Geometry: final body of the model. Coordinates: model frame, mm. A direction names the side the tool comes from. Coordinates: 2 decimals unless noted, no trailing zeros. Write each loop counter-clockwise with the first axis right and the second up, starting at its lowest first coordinate (ties: lowest second). Pieces come first, ordered by that corner, then holes. Notation, with made-up numbers: M 15,86 L 33,86 A26 ccw 33,124 Z; hole C 53,13 d8. An arc over 180 degrees is marked long. Write item = value, one per line. Start each with the question number.
Item 1: Reachability of faces 1 (the flat face through (0, 0, -9)), 2 (the cylindrical face through (-1.22, -15.16, -4.09)), 3 (the cylindrical face through (-4.09, -15.05, -1.23)), 4 (the cylindrical face through (2.26, 1.29, -1.18)), 5 (the flat face through (0, 2, -9)) from +Z, -Z, +X, -X, +Y, -Y: full face, straight path, thin tool, end or side. Return the list, or none.
Item 2: Section B-B on z = 0. Give the number of separate pieces and of enclosed holes in the cut face, plus the area to 3 significant figures.
Item 3: Ray query, L1, parallel to Y at x = -5, z = 0; L2, parallel to Z at x = 0, y = 0.9; L3, parallel to Y at x = -17.5, z = -9.5. Return the intervals inside material, ascending. Write a range as [from, to].
Item 4: Section D-D on x = 13. Output: boundary loops of the cut face in (y, z), plus the area to 3 significant figures.
Item 5: First-contact query: pin 1 Ø12 at (x, y) = (-12, -5) entering from -Z; pin 2 Ø2 at (y, z) = (-15, 0) entering from +X; pin 3 Ø5 at (x, z) = (16, 4.5) entering from +Y; pin 4 Ø13 at (x, z) = (2, 10) entering from -Y. Flat tips, straight axial feed; report the tip coordinate or a pass-through.
Item 6: Section A-A on y = -15. Output: boundary loops of the cut face in (x, z).
Item 7: Pull-direction query (Y, two-part tool) for faces 6 (the flat face through (2.4, -20, -2.4)), 7 (the cylindrical face through (0.456, 1.014, 18.595)), 8 (the flat face through (2.4, 22, -2.4)), 9 (the cylindrical face through (-4.09, 16.95, -1.23)); classes: +Y half, -Y half, draft (parallel to the pull), parting line (faces both ways), or undercut.
Item 8: Section C-C on y = -7. Output: boundary loops of the cut face in (x, z).
Autodesk Inventor part; units mm, degrees
ref_plane "Work Plane1" through (-6, 0, 0) normal (1, 0, 0) x (0, 1, 0)
ref_plane "Work Plane2" through (0, 0, -6) normal (0, 0, 1) x (1, 0, 0)
ref_plane "XZ Plane" through (0, 0, 0) normal (0, 1, 0) x (-1, 0, 0)
sketch "Sketch1" plane through (0, 0, 0) normal (0, 1, 0) x (-1, 0, 0)
  circle A0 centre (0, 0) radius 21.25
  circle A1 centre (0, 0) radius 18
  point P0 (0, 18)
  point P1 (15.4613, 9.2168)
  dimension "d0" = 42.5
  dimension "d3" = 3.25
  dimension "d4" = 59.2
extrude "Extrusion1" add sketch "Sketch1" along normal blind 2 contours A0 | A1
hole "Hole1" at (0, 0, 18) at (-15.4613, 0, 9.2168) direction (0, 1, 0) diameter 1.5 depth 8 tip angle 118
sketch "Sketch2" plane through (0, 0, 0) normal (0, -1, 0) x (1, 0, 0)
  circle A0 centre (0, 0) radius 6
  dimension "d19" = 12
extrude "Extrusion2" add sketch "Sketch2" along normal blind 20 and the other way blind 22
chamfer "Chamfer2" distance 0.5 angle 45 2 edges at (-6, 22, 0) (-6, -20, 0)
fillet "Fillet1" radius 1 2 edges at (-6, 0, 0) (-6, 2, 0)
sketch "Sketch3" plane through (0, -20, 0) normal (0, -1, 0) x (1, 0, 0)
  point P0 (0, 0)
  point P1 (0, 0)
hole "Hole3" at (0, -20, 0) direction (0, 1, 0) diameter 5.1 end through all
chamfer "Chamfer3" distance 0.5 angle 45 2 edges at (0, -20, 2.55) (0, 22, 2.55)
ref_plane "Work Plane1" through (-6, 0, 0) normal (1, 0, 0) x (0, 1, 0)
sketch "Sketch4" plane through (-6, 0, 0) normal (1, 0, 0) x (0, 1, 0)
  line L0 (22, 5.5) -> (22, -5.5)
  line L1 (-20, -5.5) -> (-20, 5.5)
  point P0 (0, 0)
  point P1 (17, 0)
  point P2 (-15, 0)
  dimension "d41" = 5
  dimension "d42" = 5
ref_plane "Work Plane2" through (0, 0, -6) normal (0, 0, 1) x (1, 0, 0)
sketch "Sketch6" plane through (0, 0, -6) normal (0, 0, 1) x (1, 0, 0)
  line L0 (5.5, -20) -> (-5.5, -20)
  line L1 (-5.5, 22) -> (5.5, 22)
  point P0 (0, 0)
  point P1 (0, -15)
  point P2 (0, 17)
  dimension "d43" = 5
  dimension "d44" = 5
hole "Hole4" at (-6, -15, 0) at (-6, 17, 0) direction (1, 0, 0) diameter 2.459 depth 5.8 tip angle 118
hole "Hole5" at (0, -15, -6) at (0, 17, -6) direction (0, 0, 1) diameter 2.459 depth 5.8 tip angle 118
properties part number "EncoderDisk"
Responses:
q1.face_1 = -Y
q1.face_2 = -Z
q1.face_3 = -X
q1.face_4 = +Y, -Y
q1.face_5 = +Y
q2.separate_pieces = 4
q2.enclosed_holes = 0
q2.area = 334 mm²
q3.L1 = [-20, -16.23], [-13.77, 15.77], [18.23, 22]
q3.L2 = [-21.25, -2.55], [2.55, 17.25], [18.75, 21.25]
q3.L3 = [0, 2]
q4.outline = M 0,-16.81 L 2,-16.81 L 2,16.81 L 0,16.81 Z
q4.area = 67.2 mm²
q5.pin_1 = -19.39
q5.pin_2 = 6
q5.pin_3 = 2
q5.pin_4 = -20
q6.outline = M -5.87,-1.23 A6 ccw -1.23,-5.87 L -1.23,-2.23 A2.55 cw -2.23,-1.23 Z; M -5.87,1.23 L -2.23,1.23 A2.55 cw long 1.23,-2.23 L 1.23,-5.87 A6 ccw long Z
q7.face_6 = -Y half
q7.face_7 = draft
q7.face_8 = +Y half
q7.face_9 = undercut
q8.outline = C 0,0 d12; hole C 0,0 d5.1
